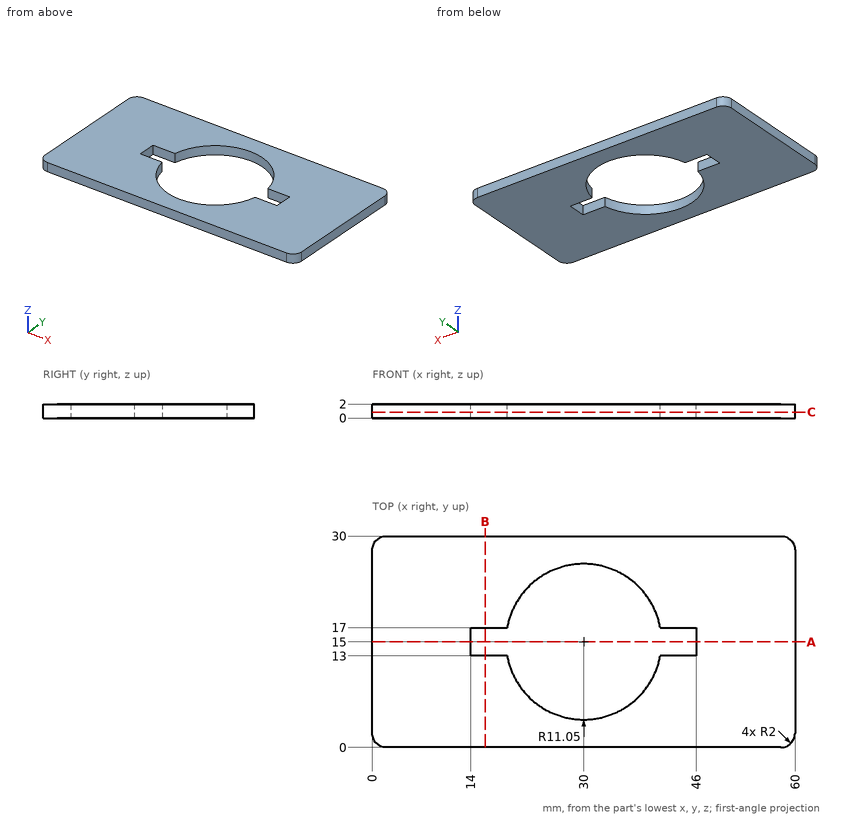
Study the drawing (mm; zero at the part's minimum x, y, z) and answer. Coordinates: 2 decimals unless noted, no trailing zeros. Loops run counter-clockwise (first coordinate to the right, second up) from the corner with the lowest first, then second, coordinate; pieces in that order, holes last. Notation, with made-up numbers: M 59,72 L 83,72 A23 cw 83,96 Z; hole C -38,-7.5 d11. An arc over 180 degrees is marked long. Answer in a Markdown table with one row per item. Add a question column.
1. Find section B-B, the plane x = 16. Write down the section's boundary in (y, z).
2. Find section A-A, the plane y = 15. Write down the section's boundary in (x, z), then the cut area to 3 significant figures.
3. Find section C-C, the plane z = 0.85. Write down the section's boundary in (x, y).
4. Consider L1, parallel to X at y = 14.75, z = 1.8; L2, parallel to Y at x = 42.5, z = 0.7; L3, parallel to Y at x = 36.5, z = 1.75. Determine where each line is inside the solid, lowest interval first.
Reported:
| question | item | result |
|---|---|---|
| 1 | outline | M 0,0 L 13,0 L 13,2 L 0,2 Z; M 17,0 L 30,0 L 30,2 L 17,2 Z |
| 2 | outline | M 0,0 L 14,0 L 14,2 L 0,2 Z; M 46,0 L 60,0 L 60,2 L 46,2 Z |
| 2 | area | 56.0 mm^2 |
| 3 | outline | M 0,2 A2 ccw 2,0 L 58,0 A2 ccw 60,2 L 60,28 A2 ccw 58,30 L 2,30 A2 ccw 0,28 Z; hole M 14,13 L 19.13,13 A11.05 ccw 40.87,13 L 46,13 L 46,17 L 40.87,17 A11.05 ccw 19.13,17 L 14,17 Z |
| 4 | L1 | x = 0 to 14, 46 to 60 |
| 4 | L2 | y = 0 to 13, 17 to 30 |
| 4 | L3 | y = 0 to 6.06, 23.94 to 30 |
